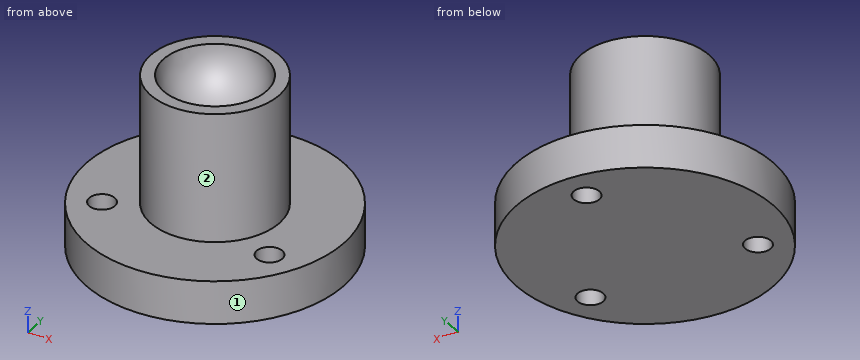
from build123d import *

# Parameters (mm, degrees)
SKETCH1_R           = 7.5
SKETCH1_R_2         = 6
BOSS_EXTRUDE1_DEPTH = 20
SKETCH1_4_R         = 6
BOSS_EXTRUDE2_DEPTH = 20
SKETCH1_5_R         = 15
SKETCH1_5_R_2       = 7.5
BOSS_EXTRUDE3_DEPTH = 5
SKETCH3_R           = 1.5
CUT_EXTRUDE1_DEPTH  = 11
SCALE1_SCALE        = 0.5
SCALE2_SCALE        = 1.25
SCALE3_SCALE        = 1.1


with BuildPart() as part:
    # Sketch1 → Boss-Extrude1 (new body)
    with BuildSketch(Plane.XY):
        Circle(SKETCH1_R)
        Circle(SKETCH1_R_2, mode=Mode.SUBTRACT)
    extrude(amount=BOSS_EXTRUDE1_DEPTH)

    # Sketch1<4> → Boss-Extrude2 (add)
    with BuildSketch(Plane.XY):
        Circle(SKETCH1_4_R)
    extrude(amount=BOSS_EXTRUDE2_DEPTH)

    # Sketch1<5> → Boss-Extrude3 (add)
    with BuildSketch(Plane.XY):
        Circle(SKETCH1_5_R)
        Circle(SKETCH1_5_R_2, mode=Mode.SUBTRACT)
    extrude(amount=BOSS_EXTRUDE3_DEPTH)

    # Sketch2 → Cut-Revolve1 (revolve, cut)
    with BuildSketch(Plane.XY.offset(20)):
        with BuildLine():
            Line((0, 6), (0, -6))
            ThreePointArc((0, -6), (6, 0), (0, 6))
        make_face()
    revolve(axis=Axis((0, 13.785304087, 20), (0, -1, 0)), mode=Mode.SUBTRACT)

    # Sketch3 → Cut-Extrude1 (cut)
    with BuildSketch(Plane.XY.offset(5)):
        with Locations((0, 11.3)):
            Circle(SKETCH3_R)
        with Locations((9.786087063, -5.65)):
            Circle(SKETCH3_R)
        with Locations((-9.786087063, -5.65)):
            Circle(SKETCH3_R)
    extrude(amount=-CUT_EXTRUDE1_DEPTH, mode=Mode.SUBTRACT)


with BuildPart() as part_1:
    # Scale1: scaled about (0, 0, 5.984924623)
    add(part.part.scale(SCALE1_SCALE).moved(Location((0, 0, 2.992462312))))


with BuildPart() as part_2:
    # Scale2: scaled about (0, 0, 5.984924623)
    add(part_1.part.scale(SCALE2_SCALE).moved(Location((0, 0, -1.496231156))))


with BuildPart() as part_3:
    # Scale3: scaled about (0, 0, 5.984924623)
    add(part_2.part.scale(SCALE3_SCALE).moved(Location((0, 0, -0.598492462))))


solid = part_3.part
Work out the finished part from the listing and answer in its coordinate system (mm). Face numbers are marked on the shaded views. A direction names the side the tool comes from. Coordinates: 2 decimals unless noted, no trailing zeros. Loops run counter-clockwise (first coordinate to the right, second up) from the corner with the lowest first, then second, coordinate; pieces in that order, holes last. Notation, with made-up numbers: M 11,57.25 L 58,57.25 A17 ccw 58,67.25 Z; hole C 6.5,69 d5. An arc over 180 degrees is marked long. Answer in a Markdown table with one row per item. Add a question column.
1. Find section C-C, the plane z = 10.75. Write down the section's boundary in (x, y), then the cut area to 3 significant figures.
2. A tool of negligible diameter and unlimited length cuts with its end or side. For the marked faces 1 and 2, from which of +Z, -Z, +X, -X, +Y, -Y can it reach the whole face along a straight path? Write none if from no direction.
3. Flat-ended cylindrical pins translate along their axes: P1, Ø5, axis at x = 6.5, z = 12, coming from the +Y side; P2, Ø1, axis at x = 2.5, z = 13.5, coming from the -Y side; P3, Ø3, axis at x = 5, z = 14, coming from the +Y side. Find the tip coordinate at first contact, or state that the pin passes through.
4. Find section D-D, the plane x = 7. Write down the section's boundary in (y, z).
5. Consider L1, parallel to Y at x = 0, z = 4.05; L2, parallel to Z at x = 5.75, y = -1.5; L3, parallel to Y at x = 1.75, z = 12.75. Determine where each line is inside the solid, lowest interval first.
Reported:
| question | item | result |
|---|---|---|
| 1 | outline | C 0,0 d10.31 |
| 1 | area | 83.5 mm^2 |
| 2 | face 1 | +Z, -Z |
| 2 | face 2 | +Z |
| 3 | P1 | stops at y = 3.25 |
| 3 | P2 | stops at y = -4.75 |
| 3 | P3 | stops at y = 3.79 |
| 4 | outline | M -7.57,1.87 L -4.88,1.87 L -4.88,5.31 L -7.57,5.31 Z; M -2.89,1.87 L 7.57,1.87 L 7.57,5.31 L -2.89,5.31 Z |
| 5 | L1 | y = -10.31 to 6.74, 8.8 to 10.31 |
| 5 | L2 | z = 1.87 to 5.31 |
| 5 | L3 | y = -4.85 to -2.39, 2.39 to 4.85 |
